Could you check a few things on this model? Use its own coordinates, in mm. Face numbers are marked on the shaded views. A direction names the side the tool comes from. Give positions to 0.01 mm unless a question says otherwise; leave off trailing zeros. Order: outer loops, then holes, each group sorted by start corner. A loop starts at its lowest first (then second) coordinate and runs counter-clockwise, first axis right, second up. Notation, with made-up numbers: M -11,-28 L 6,-28 A20 cw 6,-16 Z; hole C 46.25,16 d7. An arc over 180 degrees is marked long. Answer in a Markdown table with one row per item. Add a question column.
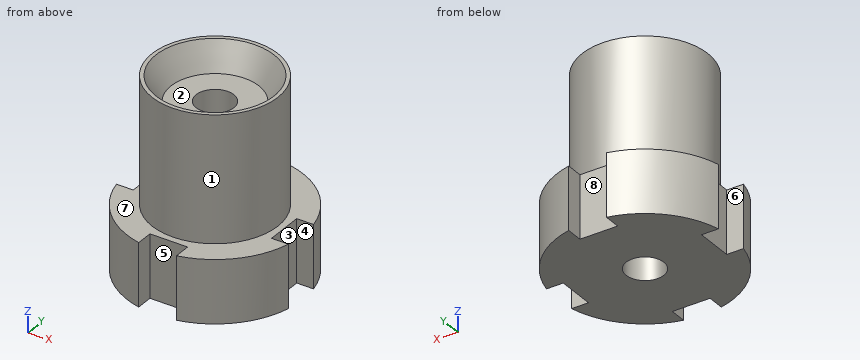
Autodesk Inventor part; units mm, degrees
ref_plane "YZ Plane" through (0, 0, 0) normal (1, 0, 0) x (0, 1, 0)
ref_plane "XZ Plane" through (0, 0, 0) normal (0, 1, 0) x (-1, 0, 0)
ref_plane "XY Plane" through (0, 0, 0) normal (0, 0, 1) x (1, 0, 0)
sketch "Sketch1" plane through (0, 0, 0) normal (0, 0, 1) x (1, 0, 0)
  circle A0 centre (0, 0) radius 7
  dimension "d0" = 14
extrude "Extrusion1" add sketch "Sketch1" along normal blind 5
sketch "Sketch2" plane through (0, 0, 5) normal (0, 0, 1) x (1, 0, 0)
  circle A0 centre (0, 0) radius 5
  dimension "d3" = 10
extrude "Extrusion2" add sketch "Sketch2" along normal blind 10
thread "Thread1"
sketch "Sketch3" plane through (0, 0, 15) normal (0, 0, 1) x (1, 0, 0)
  point P0 (0, 0)
  point P1 (0, 0)
hole "Hole1" at (0, 0, 15) direction (0, 0, -1) diameter 7 end through all
chamfer "Chamfer1" distance 1.2 angle 60 1 edges at (0, 3.5, 15) measured on face at (4.4431, -0.5395, 15)
sketch "Sketch4" plane through (0, 0, 0) normal (0, 0, -1) x (-1, 0, 0)
  circle A0 centre (0, 0) radius 1.5
  circle A1 centre (0, 0) radius 3.5
  dimension "d18" = 3
extrude "Extrusion3" add sketch "Sketch4" against normal blind 13
sketch "Sketch5" plane through (0, 0, 5) normal (0, 0, 1) x (1, 0, 0)
  circle A0 centre (0, 0) radius 7
  line L0 (-1.5, 8.5) -> (1.5, 8.5)
  line L1 (1.5, 8.5) -> (1.5, 5.5)
  line L2 (1.5, 5.5) -> (-1.5, 5.5)
  line L3 (-1.5, 5.5) -> (-1.5, 8.5)
  circle A1 centre (0, 0) radius 7
  line L4 (-1.5, 8.5) -> (1.5, 5.5) construction
  line L5 (1.5, 8.5) -> (-1.5, 5.5) construction
  line L6 (8.5, 1.5) -> (5.5, 1.5)
  line L7 (5.5, 1.5) -> (5.5, -1.5)
  line L8 (5.5, -1.5) -> (8.5, -1.5)
  line L9 (8.5, -1.5) -> (8.5, 1.5)
  line L10 (8.5, 1.5) -> (5.5, -1.5) construction
  line L11 (5.5, 1.5) -> (8.5, -1.5) construction
  line L12 (1.5, -8.5) -> (-1.5, -8.5)
  line L13 (-1.5, -8.5) -> (-1.5, -5.5)
  line L14 (-1.5, -5.5) -> (1.5, -5.5)
  line L15 (1.5, -5.5) -> (1.5, -8.5)
  line L16 (1.5, -8.5) -> (-1.5, -5.5) construction
  line L17 (-1.5, -8.5) -> (1.5, -5.5) construction
  line L18 (-8.5, 1.5) -> (-5.5, 1.5)
  line L19 (-5.5, 1.5) -> (-5.5, -1.5)
  line L20 (-5.5, -1.5) -> (-8.5, -1.5)
  line L21 (-8.5, -1.5) -> (-8.5, 1.5)
  line L22 (-8.5, 1.5) -> (-5.5, -1.5) construction
  line L23 (-5.5, 1.5) -> (-8.5, -1.5) construction
  point P0 (0, 7)
  point P1 (7, 0)
  point P2 (0, -7)
  point P3 (-7, 0)
  dimension "d21" = 3
  dimension "d22" = 3
  dimension "d23" = 3
  dimension "d24" = 3
  dimension "d25" = 3
  dimension "d26" = 3
  dimension "d27" = 3
  dimension "d28" = 3
extrude "Extrusion4" cut sketch "Sketch5" against normal blind 13 contours A0 L8 L7 L6 | A0 L6 L9 L8 | L1 L2 L3 A0 | A0 L3 L0 L1 | L15 L12 L13 A0 | A0 L13 L14 L15 | L18 L19 L20 A0 | A0 L20 L21 L18
properties part number "HUDSON-1-36"
1. For the marked faces 4, 5, 6, 7 and 8, which set-ups out of +Z, -Z, +X, -X, +Y, -Y let a thin tool reach every point of the face, with its end or its side?
2. Suppose I cut it at D-D on z = 12.5. List the corners of the cut face in (x, y) for me, plus the area to 3 significant figures.
3. Thinking about a two-plate mould opening in X: for the marked faces 1, 2 and 3, which applies, pulls with the +X half, pulls with the -X half, needs draft (parallel to the pull), parting line crosses it, or undercut?
4. Will these pins go through, and if not, where does the flat tip stop? P1, Ø1.5, axis at y = -6.5, z = 3.5, coming from the +X side; P2, Ø2.5, axis at x = 0, y = 0, coming from the +Z side; P3, Ø5, axis at y = 3, z = 13, coming from the +X side; P4, Ø1.5, axis at y = -6, z = 2.5, coming from the -X side.
5. Suppose I cut it at C-C on z = 2.5. List the corners of the cut face in (x, y) for me.
6. If I drill on line 1 along Y through (x, z) = (0, 4); line 2 along Y through (x, z) = (0, 6.5); line 3 along Z through (x, y) = (-3.25, 5.5), over which ranges is the centre line in solid material (lowest first)? Write a range as [from, to].
7. Suppose I cut it at A-A on x = 0. List the corners of the cut face in (y, z) for me, plus the area to 3 significant figures.
Findings below:
| question | item | result |
|---|---|---|
| 1 | face 4 | +Z, -Z, +X |
| 1 | face 5 | +Z, -Z, -Y |
| 1 | face 6 | +Z, -Z, -X |
| 1 | face 7 | +Z |
| 1 | face 8 | +Z, -Z, +Y |
| 2 | outline | C 0,0 d10; hole C 0,0 d3 |
| 2 | area | 71.5 mm2 |
| 3 | face 1 | parting line crosses it |
| 3 | face 2 | undercut |
| 3 | face 3 | pulls with the +X half |
| 4 | P1 | x = 3.99 |
| 4 | P2 | through |
| 4 | P3 | x = 4.97 |
| 4 | P4 | x = -4.63 |
| 5 | outline | M -6.84,-1.5 A7 ccw -1.5,-6.84 L -1.5,-5.5 L 1.5,-5.5 L 1.5,-6.84 A7 ccw 6.84,-1.5 L 5.5,-1.5 L 5.5,1.5 L 6.84,1.5 A7 ccw 1.5,6.84 L 1.5,5.5 L -1.5,5.5 L -1.5,6.84 A7 ccw -6.84,1.5 L -5.5,1.5 L -5.5,-1.5 Z; hole C 0,0 d3 |
| 6 | line 1 | [-5.5, -1.5], [1.5, 5.5] |
| 6 | line 2 | [-5, -1.5], [1.5, 5] |
| 6 | line 3 | [0, 5] |
| 7 | outline | M -5.5,0 L -1.5,0 L -1.5,13 L -3.5,13 L -3.5,12.92 L -4.7,15 L -5,15 L -5,5 L -5.5,5 Z; M 1.5,0 L 5.5,0 L 5.5,5 L 5,5 L 5,15 L 4.7,15 L 3.5,12.92 L 3.5,13 L 1.5,13 Z |
| 7 | area | 99.5 mm2 |
